The listing builds one solid part. Answer for the finished solid, in the listing's coordinates (mm). Face numbers are marked on the shaded views. A direction names the side the tool comes from. Round coordinates to 2 decimals unless told otherwise and drop trailing zeros. Loops run counter-clockwise (first coordinate to the right, second up) from the corner with the lowest first, then second, coordinate; pieces in that order, holes last. Notation, with made-up numbers: (70, -27) - (123, -27) arc R32 ccw to (123, 12) - close; hole circle Ø7 at (75, 9). An arc over 180 degrees is marked (long way). Write item = value, one per line. Start each with the question number.
1) For a pull along X with two mould halves and no side action, classify the marked faces 4, 5 and 6 as released by +X, released by -X, zero draft, split by the parting line, or undercut.
2) Section A-A, the plane x = 4.75 is taken. Determine the outline of the cut face in (y, z) (3 decimals).
3) Section C-C, the plane z = 1.3 is taken. Determine the outline of the cut face in (x, y).
4) Straight lines are drawn through the part: line 1 along Y through (x, z) = (4, 0.3); line 2 along Z through (x, y) = (2.25, 13.25); line 3 along X through (y, z) = (6.75, 3.05). For each, find the intervals that lie inside material, in ascending order.
5) A tool of negligible diameter and unlimited length cuts with its end or side. For the marked faces 1, 2 and 3, from which of +Z, -Z, +X, -X, +Y, -Y can it reach the whole face along a straight path? Write none if from no direction.
6) Given pin 1 Ø3 at (x, y) = (4.06, 11.62) entering from -Z; pin 2 Ø1.7 at (y, z) = (6.5, 3) entering from +X; pin 3 Ø1.2 at (x, z) = (4.5, 2.5) entering from -Y; pin 4 Ø0.8 at (x, z) = (4.5, 2.5) entering from +Y, each flat-ended and moving along its own axis, determine where each tip first touches the part or whether it passes through.
7) Section D-D, the plane x = 1.75 is taken. Determine the outline of the cut face in (y, z).
8) Section B-B, the plane y = 2 is taken. Determine the outline of the cut face in (x, z).
from build123d import *

# Parameters (mm, degrees)
SKETCH1_W           = 8.128
SKETCH1_H           = 14.224
BOSS_EXTRUDE1_DEPTH = 1.651
SKETCH2_W           = 2.6162
SKETCH2_H           = 3.302
BOSS_EXTRUDE2_DEPTH = 1.524
SKETCH3_R           = 1.7145
CUT_EXTRUDE1_DEPTH  = 2.651


with BuildPart() as part:
    # Sketch1 → Boss-Extrude1 (new body)
    with BuildSketch(Plane.XY):
        with Locations((4.064, 7.112)):
            Rectangle(SKETCH1_W, SKETCH1_H)
    extrude(amount=BOSS_EXTRUDE1_DEPTH)

    # Sketch2 → Boss-Extrude2 (add)
    with BuildSketch(Plane.XY.offset(1.651)):
        with Locations((4.064, 6.731)):
            Rectangle(SKETCH2_W, SKETCH2_H)
    extrude(amount=BOSS_EXTRUDE2_DEPTH)

    # Sketch3 → Cut-Extrude1 (cut, through all)
    with BuildSketch(Plane.XY.offset(1.651)):
        with Locations((4.064, 11.6205)):
            Circle(SKETCH3_R)
    extrude(amount=-CUT_EXTRUDE1_DEPTH, mode=Mode.SUBTRACT)


solid = part.part
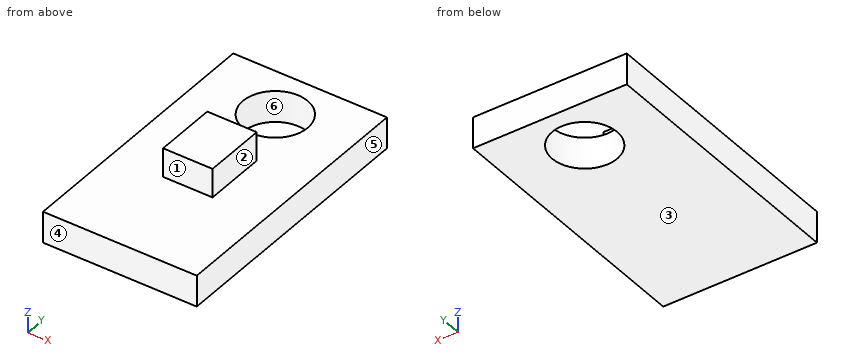
Geometry check:
q1.face_4 = zero draft
q1.face_5 = released by +X
q1.face_6 = undercut
q2.outline = (0, 0) - (10.049, 0) - (10.049, 1.651) - (8.382, 1.651) - (8.382, 3.175) - (5.08, 3.175) - (5.08, 1.651) - (0, 1.651) - close; (13.192, 0) - (14.224, 0) - (14.224, 1.651) - (13.192, 1.651) - close
q3.outline = (0, 0) - (8.13, 0) - (8.13, 14.22) - (0, 14.22) - close; hole circle Ø3.43 at (4.06, 11.62)
q4.line_1 = 0 to 9.91, 13.33 to 14.22
q4.line_2 = 0 to 1.65
q4.line_3 = 2.76 to 5.37
q5.face_1 = +Z, +X, -X, -Y
q5.face_2 = +Z, +X, +Y, -Y
q5.face_3 = -Z, +X, -X, +Y, -Y
q6.pin_1 = through
q6.pin_2 = 5.37
q6.pin_3 = 5.08
q6.pin_4 = 8.38
q7.outline = (0, 0) - (14.22, 0) - (14.22, 1.65) - (0, 1.65) - close
q8.outline = (0, 0) - (8.13, 0) - (8.13, 1.65) - (0, 1.65) - close
